```python
from build123d import *

# Parameters (mm, degrees)
F1_DEPTH = 10
F2_R     = 0.6
F3_R     = 0.3


with BuildPart() as f1:
    # F0 (on Top) → F1 (new body, symmetric)
    with BuildSketch(Plane.XY):
        Polygon((-30, 0), (0, 0), (30, 0), (30, 40), (5, 40), (8.712496, 29.8), (0, 29.8), (-8.712496, 29.8), (-5, 40), (-30, 40), align=None)
    extrude(amount=F1_DEPTH, both=True)

    # F2
    f2_edges = [f1.edges().sort_by_distance(p)[0] for p in [
        (-5, 40, 0),
        (5, 40, 0),
    ]]
    fillet(f2_edges, radius=F2_R)

    # F3
    f3_edges = [f1.edges().sort_by_distance(p)[0] for p in [
        (-8.712496, 29.8, 0),
        (8.712496, 29.8, 0),
    ]]
    fillet(f3_edges, radius=F3_R)


solid = f1.part
```
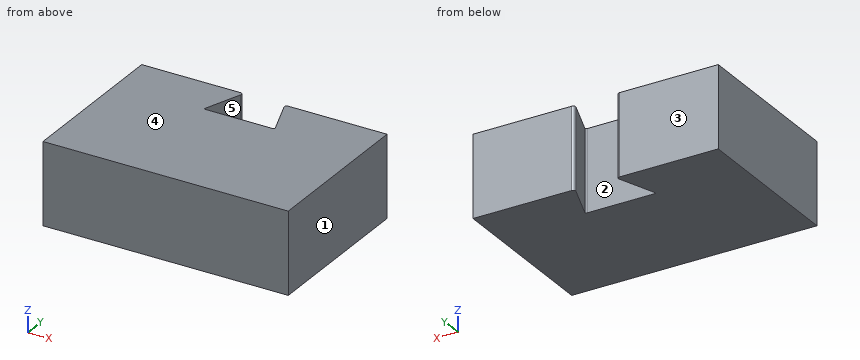
CAD build for the part. Positions are in the model's coordinates, mm. Face numbers are marked on the shaded views. A direction names the side the tool comes from. Round coordinates to 2 decimals unless told otherwise and drop trailing zeros. Loops run counter-clockwise (first coordinate to the right, second up) from the corner with the lowest first, then second, coordinate; pieces in that order, holes last. Notation, with made-up numbers: (-14.5, 64) - (9.5, 64) arc R14 cw to (9.5, 74) - close; hole circle Ø7 at (11, 84.5). An arc over 180 degrees is marked (long way). Return JSON: item names as keys, results as strings. Group by question number.
Q1. Tool access for the marked faces 4 and 5: list every direction of +Z, -Z, +X, -X, +Y, -Y with a clear straight run to the whole face (end or side of a thin tool).
Q2. Band-saw the part on C-C on x = 4. Give the cut face in (y, z), plus the area to 3 significant figures.
Q3. Two-plate mould, pull along Y, no slides. Class the marked faces 1, 2 and 3: +Y half, -Y half, draft (parallel to the pull), parting line (faces both ways), or undercut.
Q4. Band-saw the part on A-A on y = 32.5. Give the cut face in (x, z).
Q5. Band-saw the part on B-B on z = 8. Give the cut face in (x, y), plus the area to 3 significant figures.
Q6. Drill centre lines: line 1 along X through (y, z) = (30, -3.5); line 2 along X through (y, z) = (36, 3.25); line 3 along Y through (x, z) = (5, 9). Where is each one in solid material? Low to high. Write a range as [from, to].
Solutions:
{
 "1": {"face 4": "+Z, +X, -X, +Y, -Y", "face 5": "+Z, -Z"},
 "2": {"outline": "(0, -10) - (29.8, -10) - (29.8, 10) - (0, 10) - close", "area": "596 mm^2"},
 "3": {"face 1": "draft", "face 2": "undercut", "face 3": "+Y half"},
 "4": {"outline": "(-30, -10) - (-7.73, -10) - (-7.73, 10) - (-30, 10) - close; (7.73, -10) - (30, -10) - (30, 10) - (7.73, 10) - close"},
 "5": {"outline": "(-30, 0) - (30, 0) - (30, 40) - (5.86, 40) arc R0.6 ccw to (5.29, 39.19) - (8.57, 30.2) arc R0.3 cw to (8.28, 29.8) - (-8.28, 29.8) arc R0.3 cw to (-8.57, 30.2) - (-5.29, 39.19) arc R0.6 ccw to (-5.86, 40) - (-30, 40) - close", "area": "2,260 mm^2"},
 "6": {"line 1": "x = [-30, -8.57], [8.57, 30]", "line 2": "x = [-30, -6.46], [6.46, 30]", "line 3": "y = [0, 29.8]"}
}
